from build123d import *


with BuildPart() as f1:
    # F0 (on Right) → F1 (revolve)
    with BuildSketch(Plane.YZ):
        with BuildLine():
            Line((0, 28.671082), (0, 5.059838))
            Line((0, 5.059838), (7.62, 5.059838))
            Line((7.62, 5.059838), (7.62, 5.024209))
            Line((7.62, 5.024209), (17.62, 5.024209))
            Line((17.62, 5.024209), (17.62, 7.564209))
            Line((17.62, 7.564209), (7.62, 7.564209))
            Line((7.62, 7.564209), (7.62, 22.591082))
            ThreePointArc((7.62, 22.591082), (7.912893, 23.298189), (8.62, 23.591082))
            Line((8.62, 23.591082), (32, 23.591082))
            Line((32, 23.591082), (32, 28.671082))
            Line((32, 28.671082), (0, 28.671082))
        make_face()
    revolve(axis=Axis((0, -0.662774, 0), (0, 1, 0)))


solid = f1.part
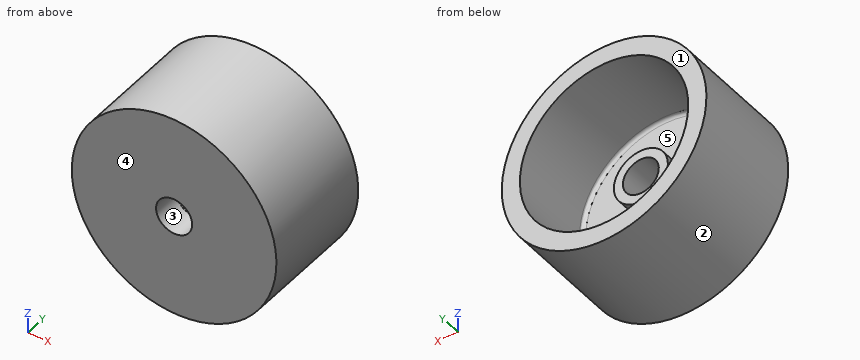
Here's how the part is built. I have some questions about the finished solid (model axes, mm). Face numbers are marked on the shaded views. A direction names the side the tool comes from. Coordinates: 2 decimals unless noted, no trailing zeros. Order: outer loops, then holes, each group sorted by start corner. A loop starts at its lowest first (then second) coordinate and runs counter-clockwise, first axis right, second up. Notation, with made-up numbers: (29.5, 9.25) - (60.5, 9.25) arc R18 ccw to (60.5, 25.25) - close; hole circle Ø5 at (69.5, 33). An arc over 180 degrees is marked (long way). Use CSV: the item, a comma, the result in double quotes. Start each with the question number.
1. Suppose I cut it at B-B on y = 14.5. List the corners of the cut face in (x, z) for me.
2. Please list where these lines run through material, in increasing order: line 1 (X direction, y = 14, z = 0); line 2 (Z direction, x = -5.5, y = 11); line 3 (Y direction, x = -12, z = 0). Write a range as from..to.
3. For the marked faces 4 and 5, which set-ups out of +Z, -Z, +X, -X, +Y, -Y let a thin tool reach every point of the face, with its end or its side?
4. Suppose I cut it at D-D on y = 22.5. List the corners of the cut face in (x, z) for me, then the cut area to 3 significant figures.
5. If we mould it in two halves opening along Z, with no side actions, what happens to the marked faces 1, 2 and 3? For each: +Z half, -Z half, draft (parallel to the pull), parting line (faces both ways), or undercut.
6. I'm going to push flat-ended pins straight in: pin 1 (4 mm diameter, centred on y = 8.5, z = -17, fed in from -X); pin 2 (11 mm diameter, centred on x = 0.5, z = 0, fed in from -Y); pin 3 (1.5 mm diameter, centred on x = -2, y = 6, fed in from -Z); pin 4 (6 mm diameter, centred on y = 9.5, z = 22, fed in from -X). Where does each tip first touch, or does it pass through?
Output:
1,outline,"circle Ø57.34 at (0, 0); circle Ø15.13 at (0, 0); hole circle Ø47.18 at (0, 0); hole circle Ø10.05 at (0, 0)"
2,line 1,"x = -28.67..-23.59, -7.56..-5.02, 5.02..7.56, 23.59..28.67"
2,line 2,"z = -28.14..-22.94, -5.19..5.19, 22.94..28.14"
2,line 3,"y = 0..7.62"
3,face 4,"+Z, -Z, +X, -X, -Y"
3,face 5,"+Y"
4,outline,"circle Ø57.34 at (0, 0); hole circle Ø47.18 at (0, 0)"
4,area,"834 mm2"
5,face 1,"draft"
5,face 2,"parting line"
5,face 3,"undercut"
6,pin 1,"stops at x = -24.43"
6,pin 2,"stops at y = 0"
6,pin 3,"stops at z = -28.64"
6,pin 4,"stops at x = -21.47"
